Could you check a few things on this model? Use its own coordinates, in mm. A direction names the side the tool comes from. Give positions to 0.01 mm unless a question says otherwise; leave off trailing zeros. Order: outer loops, then holes, each group sorted by start corner. A loop starts at its lowest first (then second) coordinate and runs counter-clockwise, first axis right, second up. Notation, with made-up numbers: (23.25, 0.25) - (63.25, 0.25) arc R8 cw to (63.25, 7.25) - close; hole circle Ø4 at (30.25, 64.25). An arc over 180 degrees is marked (long way). One line per question, with ' | ' between items. Start each with the question number.
1. Imagine slicing it at B-B (z = 13). Please give me the cut outline in (x, y), and give its area (3 significant figures).
2. Imagine slicing it at C-C (x = 18). Please give me the cut outline in (y, z).
3. If we mould it in two halves opening along X, with no side actions, what happens to faces 3 (the flat face through (88, 26, 23.812)), 4 (the flat face through (177.8, 23, 24)), 5 (the cylindrical face through (138.925, 10.239, 0.783))? For each: released by +X, released by -X, zero draft, split by the parting line, or undercut.
4. Which directions (+Z, -Z, +X, -X, +Y, -Y) give clear straight access to the entire face, cutting with the end or side of a thin tool? Please do faces 1 (the flat face through (88, 1.588, 13)), 2 (the cylindrical face through (49.334, 27.26, 24.595)).
5. Imagine slicing it at A-A (x = 63.5). Please give me the cut outline in (y, z), and give its area (3 significant figures).
6. I need wall thicknesses on probe 1 along Z at (x, y) = (16.5, 33.5); probe 2 along X at (y, z) = (25.4, 1.25); probe 3 along X at (y, z) = (12.7, 0.5). Which ranges of each line are inside material? Lowest first, please. Write a range as from..to.
7. Imagine slicing it at D-D (y = 22). Please give me the cut outline in (x, z), and give its area (3 significant figures).
Autodesk Inventor part; units mm, degrees
ref_plane "YZ Plane" through (0, 0, 0) normal (1, 0, 0) x (0, 1, 0)
ref_plane "XZ Plane" through (0, 0, 0) normal (0, 1, 0) x (-1, 0, 0)
ref_plane "XY Plane" through (0, 0, 0) normal (0, 0, 1) x (1, 0, 0)
sketch "Sketch1" plane through (0, 0, 0) normal (0, 0, 1) x (1, 0, 0)
  line L0 (0, 0) -> (177.8, 0)
  line L1 (177.8, 0) -> (177.8, 50.8)
  line L2 (177.8, 50.8) -> (0, 50.8)
  line L3 (0, 50.8) -> (0, 0)
  dimension "d0" = 177.8
  dimension "d1" = 50.8
extrude "Extrusion1" add sketch "Sketch1" along normal blind 25.4
shell "Shell1" thickness 1.5875 removed faces 2 at (0, 33.8667, 16.9333) at (177.8, 16.9333, 16.9333)
sketch "Sketch2" plane through (0, 0, 25.4) normal (0, 0, 1) x (1, 0, 0)
  line L0 (0, 0) -> (63.5, 0) construction
  line L1 (63.5, 0) -> (63.5, 25.4) construction
  line L2 (63.5, 25.4) -> (0, 25.4) construction
  line L3 (0, 25.4) -> (0, 0) construction
  dimension "d5" = 63.5
  dimension "d13" = 25.4
hole "Hole1" at (63.5, 25.4, 25.4) direction (0, 0, -1) diameter 28.575 end through all
hole "Hole2" at (12.7, 12.7, 25.4) direction (0, 0, -1) diameter 5.1594 end through all
hole "Hole3" at (38.1, 12.7, 25.4) direction (0, 0, -1) diameter 5.1594 end through all
hole "Hole4" at (165.1, 12.7, 25.4) direction (0, 0, -1) diameter 5.1594 end through all
hole "Hole5" at (139.7, 12.7, 25.4) direction (0, 0, -1) diameter 5.1594 end through all
properties part number "1x2 5 in Beam Flywheel Mount"
Results found:
1) outline: (0, 0) - (177.8, 0) - (177.8, 1.59) - (0, 1.59) - close; (0, 49.21) - (177.8, 49.21) - (177.8, 50.8) - (0, 50.8) - close | area: 565 mm2
2) outline: (0, 0) - (50.8, 0) - (50.8, 25.4) - (0, 25.4) - close; hole (1.59, 1.59) - (49.21, 1.59) - (49.21, 23.81) - (1.59, 23.81) - close
3) face 3: zero draft | face 4: released by +X | face 5: undercut
4) face 1: +X, -X | face 2: +Z, -Z
5) outline: (0, 0) - (11.11, 0) - (11.11, 1.59) - (1.59, 1.59) - (1.59, 23.81) - (11.11, 23.81) - (11.11, 25.4) - (0, 25.4) - close; (39.69, 0) - (50.8, 0) - (50.8, 25.4) - (39.69, 25.4) - (39.69, 23.81) - (49.21, 23.81) - (49.21, 1.59) - (39.69, 1.59) - close | area: 141 mm2
6) probe 1: z = 0..1.59, 23.81..25.4 | probe 2: x = 0..49.21, 77.79..177.8 | probe 3: x = 0..10.12, 15.28..35.52, 40.68..56.95, 70.05..137.12, 142.28..162.52, 167.68..177.8
7) outline: (0, 0) - (49.62, 0) - (49.62, 1.59) - (0, 1.59) - close; (0, 23.81) - (49.62, 23.81) - (49.62, 25.4) - (0, 25.4) - close; (77.38, 0) - (177.8, 0) - (177.8, 1.59) - (77.38, 1.59) - close; (77.38, 23.81) - (177.8, 23.81) - (177.8, 25.4) - (77.38, 25.4) - close | area: 476 mm2
